Input: part model. Units: mm. Frame: model coordinates. Coordinates: 2 decimals unless noted, no trailing zeros. Write each loop counter-clockwise with the first axis right and the second up, starting at its lowest first coordinate (ties: lowest second). Pieces come first, ordered by that corner, then holes. Notation, with made-up numbers: (-19, 33.25) -> (-14, 33.25) arc R25 cw to (-14, 62.25) -> close; hole circle Ø7 at (-18, 86). An arc over 180 degrees is marked (long way). Use one line per item in the form item = value. Start each with the question number.
(1) Cut plane C-C on z = -14.5. Return the cut outline in (x, y).
(2) Cut plane B-B on y = 0.9. State how many separate pieces and enclosed holes the cut face has, plus the area to 3 significant figures.
(3) Cut plane D-D on x = 11. Return the cut outline in (y, z).
(4) First-contact query: pin 1 (1.2 mm diameter, centred on x = 16.5, y = 1.5, fed in from -Z); pin 2 (2 mm diameter, centred on x = -18, y = 2, fed in from +Z); pin 3 (2 mm diameter, centred on y = 2.5, z = 18.5, fed in from +X). Flat tips, straight axial feed; report the tip coordinate or a pass-through.
(5) Ray query, line 1 along Z through (x, y) = (16, 1.2); line 2 along X through (y, z) = (3.55, -7); line 3 along X through (y, z) = (1.4, -17). Return the intervals inside material, ascending.
(6) Cut plane A-A on z = 8. Return the cut outline in (x, y), plus the area to 3 significant figures.
```python
from build123d import *

# Parameters (mm, degrees)
BOSS_EXTRUDE1_DEPTH = 4


with BuildPart() as part:
    # Sketch1 → Boss-Extrude1 (new body)
    with BuildSketch(Plane(origin=(0, 0, 0), x_dir=(1, 0, 0), z_dir=(0, 1, 0))):
        Polygon((-5, 26), (5, 26), (5, 30), (15, 30), (15, 26), (19, 26), (19, 18), (15, 18), (15, 10), (19, 10), (19, 2), (15, 2), (15, -6), (19, -6), (19, -14), (15, -14), (15, -22), (19, -22), (19, -30), (15, -30), (6, -30), (6, -36), (-6, -36), (-6, -30), (-15, -30), (-19, -30), (-19, -22), (-15, -22), (-15, -14), (-19, -14), (-19, -6), (-15, -6), (-15, 2), (-19, 2), (-19, 10), (-15, 10), (-15, 18), (-19, 18), (-19, 26), (-15, 26), (-15, 30), (-5, 30), align=None)
        with BuildLine():
            Line((-8, -18), (-8, 18))
            ThreePointArc((-8, 18), (-6, 20), (-4, 18))
            Line((-4, 18), (-4, -18))
            ThreePointArc((-4, -18), (-6, -20), (-8, -18))
        make_face(mode=Mode.SUBTRACT)
        with BuildLine():
            Line((8, -18), (8, 18))
            ThreePointArc((8, 18), (6, 20), (4, 18))
            Line((4, 18), (4, -18))
            ThreePointArc((4, -18), (6, -20), (8, -18))
        make_face(mode=Mode.SUBTRACT)
    extrude(amount=BOSS_EXTRUDE1_DEPTH)


solid = part.part
```
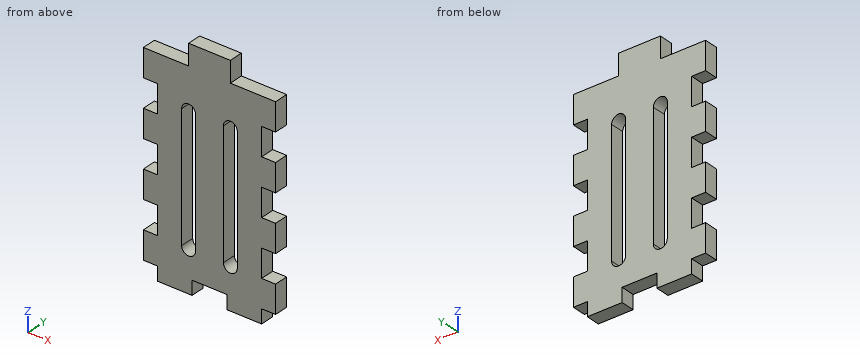
Values:
q1.outline = (-15, 0) -> (-8, 0) -> (-8, 4) -> (-15, 4) -> close; (-4, 0) -> (4, 0) -> (4, 4) -> (-4, 4) -> close; (8, 0) -> (15, 0) -> (15, 4) -> (8, 4) -> close
q2.separate_pieces = 1
q2.enclosed_holes = 2
q2.area = 1,770 mm2
q3.outline = (0, -30) -> (4, -30) -> (4, 30) -> (0, 30) -> close
q4.pin_1 = -26
q4.pin_2 = 30
q4.pin_3 = 15
q5.line_1 = -26 to -18, -10 to -2, 6 to 14, 22 to 30
q5.line_2 = -19 to -8, -4 to 4, 8 to 19
q5.line_3 = -15 to -8, -4 to 4, 8 to 15
q6.outline = (-19, 0) -> (-8, 0) -> (-8, 4) -> (-19, 4) -> close; (-4, 0) -> (4, 0) -> (4, 4) -> (-4, 4) -> close; (8, 0) -> (19, 0) -> (19, 4) -> (8, 4) -> close
q6.area = 120 mm2
